Geometry: final body of the model. Coordinates: model frame, mm. A direction names the side the tool comes from. Give positions to 0.01 mm unless a question says otherwise; leave off trailing zeros. Order: outer loops, then holes, each group sorted by start corner. A loop starts at its lowest first (then second) coordinate and runs counter-clockwise, first axis right, second up. Notation, with made-up numbers: (-13, -38) -> (44, -38) arc R30 cw to (44, 1) -> close; hole circle Ø3 at (13.25, 2). An arc over 180 degrees is marked (long way). Write item = value, one per line.
Autodesk Inventor part; units mm, degrees
ref_plane "YZ Plane" through (0, 0, 0) normal (1, 0, 0) x (0, 1, 0)
ref_plane "XZ Plane" through (0, 0, 0) normal (0, 1, 0) x (-1, 0, 0)
ref_plane "XY Plane" through (0, 0, 0) normal (0, 0, 1) x (1, 0, 0)
sketch "Esboço1" plane through (0, 0, 0) normal (0, 0, 1) x (1, 0, 0)
  line L0 (0, 0) -> (-5, 0)
  line L1 (-5, 0) -> (-5, -5)
  line L2 (-5, -5) -> (-2, -5)
  line L3 (-2, -5) -> (-2, -15)
  line L4 (-2, -15) -> (-5, -15)
  line L5 (-5, -15) -> (-5, -20)
  line L6 (-5, -20) -> (0, -20)
  line L7 (0, -20) -> (0, -17)
  line L8 (0, -17) -> (10, -17)
  line L9 (10, -17) -> (10, -20)
  line L10 (10, -20) -> (15, -20)
  line L11 (15, -20) -> (15, -15)
  line L12 (15, -15) -> (12, -15)
  line L13 (12, -15) -> (12, -5)
  line L14 (12, -5) -> (15, -5)
  line L15 (15, -5) -> (15, 0)
  line L16 (15, 0) -> (10, 0)
  line L17 (10, 0) -> (10, -3)
  line L18 (10, -3) -> (0, -3)
  line L19 (0, -3) -> (0, 0)
  dimension "d4" = 5
  dimension "d5" = 5
  dimension "d6" = 3
  dimension "d7" = 10
  dimension "d8" = 3
  dimension "d9" = 5
  dimension "d10" = 5
  dimension "d11" = 3
  dimension "d12" = 10
  dimension "d13" = 5
  dimension "d14" = 5
  dimension "d15" = 3
  dimension "d16" = 10
  dimension "d17" = 3
  dimension "d18" = 5
  dimension "d19" = 3
  dimension "d20" = 10
extrude "Extrusão1" add sketch "Esboço1" along normal blind 150
properties part number "Viga Projeto Bosch"
1) Section query B-B (z = 63). Output: boundary loops of the cut face in (x, y).
Check sheet entries:
outline = (-5, -20) -> (0, -20) -> (0, -17) -> (10, -17) -> (10, -20) -> (15, -20) -> (15, -15) -> (12, -15) -> (12, -5) -> (15, -5) -> (15, 0) -> (10, 0) -> (10, -3) -> (0, -3) -> (0, 0) -> (-5, 0) -> (-5, -5) -> (-2, -5) -> (-2, -15) -> (-5, -15) -> close
2) Section query A-A (y = -1.5). Output: boundary loops of the cut face in (x, z), plus the area to 3 significant figures.
Check sheet entries:
outline = (-5, 0) -> (0, 0) -> (0, 150) -> (-5, 150) -> close; (10, 0) -> (15, 0) -> (15, 150) -> (10, 150) -> close
area = 1,500 mm²
3) Mould query, pull axis Y, two halves, no side actions, for faces 1 (the face through (12, -20, 74)), 2 (the face through (10, -18, 74)), 3 (the face through (14, -15, 74)). Classes: +Y half, -Y half, draft (parallel to the pull), parting line (faces both ways), or undercut.
Check sheet entries:
face_1 = -Y half
face_2 = draft
face_3 = undercut
4) Line query: line 1 (Y direction, x = 13, z = 142.5); line 2 (X direction, y = -18.5, z = 31.5); line 3 (Y direction, x = 3.25, z = 38.5). Output: solid intervals per line, ascending. Write a range as from..to.
Check sheet entries:
line_1 = -20..-15, -5..0
line_2 = -5..0, 10..15
line_3 = -17..-3
5) Section query D-D (x = 4). Output: boundary loops of the cut face in (y, z), plus the area to 3 significant figures.
Check sheet entries:
outline = (-17, 0) -> (-3, 0) -> (-3, 150) -> (-17, 150) -> close
area = 2,100 mm²
6) Reachability of faces 4 (the face through (13, -5, 74)), 5 (the face through (-3, -15, 74)), 6 (the face through (0, -2, 74)), 7 (the face through (5, -17, 74)) from +Z, -Z, +X, -X, +Y, -Y: full face, straight path, thin tool, end or side. Return the list, or none.
Check sheet entries:
face_4 = +Z, -Z, +X
face_5 = +Z, -Z, -X
face_6 = +Z, -Z, +Y
face_7 = +Z, -Z, -Y
7) Section query C-C (y = -8.25). Output: boundary loops of the cut face in (x, z).
Check sheet entries:
outline = (-2, 0) -> (12, 0) -> (12, 150) -> (-2, 150) -> close
8) First-contact query: P1, Ø1.5, axis at y = -12, z = 97, coming from the -X side; P2, Ø5, axis at x = 4, z = 41.5, coming from the -Y side. Flat tips, straight axial feed; report the tip coordinate or a pass-through.
Check sheet entries:
P1 = -2
P2 = -17
